```python
from build123d import *

# Parameters (mm, degrees)
SKETCH1_W          = 3
SKETCH1_H          = 14
BASE_EXTRUDE_DEPTH = 3


with BuildPart() as part:
    # Sketch1 → Base-Extrude (new body)
    with BuildSketch(Plane.XY):
        with BuildLine():
            Line((-1033.116910611, 53.997744838), (-1033.116910611, 44.593073912))
            Line((-1033.116910611, 44.593073912), (-1034.65769353, 44.593073912))
            Line((-1034.65769353, 44.593073912), (-1034.65769353, 39.402415763))
            Line((-1034.65769353, 39.402415763), (-1033.116910611, 39.402415763))
            Line((-1033.116910611, 39.402415763), (-1033.116910611, 29.997744838))
            ThreePointArc((-1033.116910611, 29.997744838), (-1033.702697049, 28.583531275), (-1035.116910611, 27.997744838))
            Line((-1035.116910611, 27.997744838), (-1041.116910611, 27.997744838))
            Line((-1041.116910611, 27.997744838), (-1041.116910611, 29.997744838))
            Line((-1041.116910611, 29.997744838), (-1042.616910611, 29.997744838))
            Line((-1042.616910611, 29.997744838), (-1044.116910611, 29.997744838))
            Line((-1044.116910611, 29.997744838), (-1044.116910611, 27.997744838))
            Line((-1044.116910611, 27.997744838), (-1050.116910611, 27.997744838))
            ThreePointArc((-1050.116910611, 27.997744838), (-1051.531124173, 28.583531275), (-1052.116910611, 29.997744838))
            Line((-1052.116910611, 29.997744838), (-1052.116910611, 39.402415763))
            Line((-1052.116910611, 39.402415763), (-1049.190418334, 39.402415763))
            Line((-1049.190418334, 39.402415763), (-1049.190418334, 44.593073912))
            Line((-1049.190418334, 44.593073912), (-1052.116910611, 44.593073912))
            Line((-1052.116910611, 44.593073912), (-1052.116910611, 53.997744838))
            ThreePointArc((-1052.116910611, 53.997744838), (-1051.531124173, 55.4119584), (-1050.116910611, 55.997744838))
            Line((-1050.116910611, 55.997744838), (-1044.116910611, 55.997744838))
            Line((-1044.116910611, 55.997744838), (-1044.116910611, 53.997744838))
            Line((-1044.116910611, 53.997744838), (-1042.616910611, 53.997744838))
            Line((-1042.616910611, 53.997744838), (-1041.116910611, 53.997744838))
            Line((-1041.116910611, 53.997744838), (-1041.116910611, 55.997744838))
            Line((-1041.116910611, 55.997744838), (-1035.116910611, 55.997744838))
            ThreePointArc((-1035.116910611, 55.997744838), (-1033.702697049, 55.4119584), (-1033.116910611, 53.997744838))
        make_face()
        with Locations((-1042.616910611, 41.997744838)):
            Rectangle(SKETCH1_W, SKETCH1_H, mode=Mode.SUBTRACT)
    extrude(amount=BASE_EXTRUDE_DEPTH)


solid = part.part
```
For this review, take the finished solid that the model builds, in its own axes (mm). A direction names the side the tool comes from. Coordinates: 2 decimals unless noted, no trailing zeros. Loops run counter-clockwise (first coordinate to the right, second up) from the corner with the lowest first, then second, coordinate; pieces in that order, holes last. Notation, with made-up numbers: (39.5, 67.5) -> (50.5, 67.5) arc R16 cw to (50.5, 92.5) -> close; hole circle Ø3 at (79.5, 78). An arc over 180 degrees is marked (long way). Return JSON: item names as keys, results as strings. Group by question number.
(1) Consider section B-B, the plane x = -1041.75. Give the boundary of the cut face in (y, z).
(2) Consider section A-A, the plane y = 45.75. Give the boundary of the cut face in (x, z).
(3) Tool access review of faces 1 (the flat face through (-1051, 39.402, 1)), 2 (the flat face through (-1043, 48.998, 1)), 3 (the flat face through (-1043, 53.998, 1)), 4 (the cylindrical face through (-1051.52, 28.57, 1.48)), 5 (the flat face through (-1038, 27.998, 1)): name each direction out of +Z, -Z, +X, -X, +Y, -Y from which nothing blocks a thin tool from reaching the whole face with its end or side.
(4) For pin 1 Ø1.5 at (x, z) = (-1042.5, 1.5) entering from -Y; pin 2 Ø1.5 at (y, z) = (41.5, 1) entering from -X; pin 3 Ø1 at (y, z) = (55.5, 2) entering from +X, all flat-tipped, find the tip position at first contact; note any pin that passes through.
(5) Consider section C-C, the plane z = 0.5. Give the boundary of the cut face in (x, y).
(6) Mouldability with a two-part tool opening along X and no side actions: class faces 6 (the flat face through (-1041.117, 29, 1)), 7 (the flat face through (-1034, 44.593, 1)), 8 (the flat face through (-1033.117, 35, 1)) as pulls with the +X half, pulls with the -X half, needs draft (parallel to the pull), parting line crosses it, or undercut.
(7) To check wall thickness, follow L1, parallel to X at y = 43, z = 1.45; L2, parallel to X at y = 48.75, z = 1.25; L3, parallel to Y at x = -1050, z = 1.2. State the ranges of each line that lie inside material, in increasing order.
Results below:
{
 "1": {"outline": "(30, 0) -> (35, 0) -> (35, 3) -> (30, 3) -> close; (49, 0) -> (54, 0) -> (54, 3) -> (49, 3) -> close"},
 "2": {"outline": "(-1052.12, 0) -> (-1044.12, 0) -> (-1044.12, 3) -> (-1052.12, 3) -> close; (-1041.12, 0) -> (-1033.12, 0) -> (-1033.12, 3) -> (-1041.12, 3) -> close"},
 "3": {"face 1": "+Z, -Z, -X", "face 2": "+Z, -Z", "face 3": "+Z, -Z, +Y", "face 4": "+Z, -Z, -X, -Y", "face 5": "+Z, -Z, +X, -X, -Y"},
 "4": {"pin 1": "stops at y = 30", "pin 2": "stops at x = -1049.19", "pin 3": "stops at x = -1033.39"},
 "5": {"outline": "(-1052.12, 30) arc R2 ccw to (-1050.12, 28) -> (-1044.12, 28) -> (-1044.12, 30) -> (-1041.12, 30) -> (-1041.12, 28) -> (-1035.12, 28) arc R2 ccw to (-1033.12, 30) -> (-1033.12, 39.4) -> (-1034.66, 39.4) -> (-1034.66, 44.59) -> (-1033.12, 44.59) -> (-1033.12, 54) arc R2 ccw to (-1035.12, 56) -> (-1041.12, 56) -> (-1041.12, 54) -> (-1044.12, 54) -> (-1044.12, 56) -> (-1050.12, 56) arc R2 ccw to (-1052.12, 54) -> (-1052.12, 44.59) -> (-1049.19, 44.59) -> (-1049.19, 39.4) -> (-1052.12, 39.4) -> close; hole (-1044.12, 35) -> (-1041.12, 35) -> (-1041.12, 49) -> (-1044.12, 49) -> close"},
 "6": {"face 6": "undercut", "face 7": "needs draft", "face 8": "pulls with the +X half"},
 "7": {"L1": "x = -1049.19 to -1044.12, -1041.12 to -1034.66", "L2": "x = -1052.12 to -1044.12, -1041.12 to -1033.12", "L3": "y = 28 to 39.4, 44.59 to 56"}
}
